```python
from build123d import *

# Parameters (mm, degrees)
SKETCH5_R           = 37.8968
BOSS_EXTRUDE2_DEPTH = 19.05
CUT_EXTRUDE1_DEPTH  = 22.05
CIRPATTERN1_COUNT   = 25
SKETCH9_R           = 7.25
CUT_EXTRUDE2_DEPTH  = 25.4


with BuildPart() as part:
    # Sketch5 → Boss-Extrude2 (new body)
    with BuildSketch(Plane(origin=(0, 0, 0), x_dir=(1, 0, 0), z_dir=(0, 1, 0))):
        with Locations(Location((0, 0, 0), (0, 0, 90))):
            Circle(SKETCH5_R)
    extrude(amount=BOSS_EXTRUDE2_DEPTH)

    # Sketch8 → Cut-Extrude1 (cut)
    with BuildSketch(Plane(origin=(0, 19.05, 0), x_dir=(1, 0, 0), z_dir=(0, 1, 0))):
        Polygon((0, 37.8968), (2.36, 37.8968), (1.66, 35.8968), (0, 35.8968), (-1.66, 35.8968), (-2.36, 37.8968), align=None)
    cut_extrude1 = extrude(amount=-CUT_EXTRUDE1_DEPTH, mode=Mode.SUBTRACT)

    # CirPattern1: Cut-Extrude1 ×25 about axis
    cirpattern1_axis = Axis((0, 0, 0), (0, 1, 0))
    for i in range(1, CIRPATTERN1_COUNT):
        add(cut_extrude1.rotate(cirpattern1_axis, i * 360 / CIRPATTERN1_COUNT), mode=Mode.SUBTRACT)

    # Sketch9 → Cut-Extrude2 (cut)
    with BuildSketch(Plane(origin=(0, 19.05, 0), x_dir=(1, 0, 0), z_dir=(0, 1, 0))):
        Circle(SKETCH9_R)
        Polygon((2.6, 9.75), (2.6, 7.25), (0, 7.25), (-2.6, 7.25), (-2.6, 9.75), align=None)
        with BuildLine():
            ThreePointArc((-2.6, 6.767754428), (-1.32217253, 7.128419166), (0, 7.25))
            Line((0, 7.25), (-2.6, 7.25))
            Line((-2.6, 7.25), (-2.6, 6.767754428))
        make_face()
        with BuildLine():
            Line((2.6, 7.25), (0, 7.25))
            ThreePointArc((0, 7.25), (1.32217253, 7.128419166), (2.6, 6.767754428))
            Line((2.6, 6.767754428), (2.6, 7.25))
        make_face()
    extrude(amount=-CUT_EXTRUDE2_DEPTH, mode=Mode.SUBTRACT)


solid = part.part
```
For this review, take the finished solid that the model builds, in its own axes (mm). A direction names the side the tool comes from. Coordinates: 2 decimals unless noted, no trailing zeros. Order: outer loops, then holes, each group sorted by start corner. A loop starts at its lowest first (then second) coordinate and runs counter-clockwise, first axis right, second up. Notation, with made-up numbers: (41, 57.5) -> (56, 57.5) arc R36 cw to (56, 91.5) -> close; hole circle Ø9 at (76, -1). An arc over 180 degrees is marked (long way). Use CSV: the item, a comma, the result in double quotes. Start each with the question number.
Item 1: Draft analysis for pull direction X (two halves, no side actions). For faces 1 (the face through (-21.081, 9.658, 29.055)), 2 (the face through (-7.23, 9.66, -36.21)), 3 (the face through (-32, 9.4, 20.3)), 4 (the face through (37.82, 9.39, 2.41)), state which applies: pulls with the +X half, pulls with the -X half, needs draft (parallel to the pull), parting line crosses it, or undercut.
Item 2: We need section A-A, the plane x = 0. Give the boundary of the cut face in (y, z).
Item 3: We need section B-B, the plane z = -23.5. Give the boundary of the cut face in (x, y), then the cut area to 3 significant figures.
Item 4: Wall thickness on probe 1 along Z at (x, y) = (0, 10.5); probe 2 along X at (y, z) = (5.25, 0); probe 3 along Z at (x, y) = (3, 13.25): over which ranges is each line inside the solid? List them lowest first.
Item 5: Insertion check: pin 1 (5 mm diameter, centred on y = 16.5, z = 12, fed in from -X); pin 2 (4 mm diameter, centred on x = -1, y = 11, fed in from +Z); pin 3 (1.5 mm diameter, centred on x = 7.5, y = 2.5, fed in from +Z). Each pin has a flat end and moves straight along its axis. Give the tip position at first contact, or say it passes through.
Item 6: For faces 5 (the face through (-26.68, 9.66, -25.5)), 6 (the face through (35.265, 9.658, 6.704)), 7 (the face through (4.783, 9.392, -37.594)), 8 (the face through (9.392, 9.392, 36.715)), 9 (the face through (-36.596, 9.658, 4.943)), list the 3-axis set-ups (+Z, -Z, +X, -X, +Y, -Y) from which the entire face can be reached by the end or side of a thin tool; tool diameter is ignored.
Item 7: We need section C-C, the plane x = 13.5. Give the boundary of the cut face in (y, z), then the cut area to 3 significant figures.
Derived:
1,face 1,"undercut"
1,face 2,"undercut"
1,face 3,"pulls with the -X half"
1,face 4,"pulls with the +X half"
2,outline,"(0, -35.9) -> (19.05, -35.9) -> (19.05, -9.75) -> (0, -9.75) -> close; (0, 7.25) -> (19.05, 7.25) -> (19.05, 37.9) -> (0, 37.9) -> close"
3,outline,"(-29.73, 0) -> (29.73, 0) -> (29.73, 19.05) -> (-29.73, 19.05) -> close"
3,area,"1,130 mm^2"
4,probe 1,"z = -35.9 to -9.75, 7.25 to 37.9"
4,probe 2,"x = -37.9 to -7.25, 7.25 to 37.9"
4,probe 3,"z = -37.78 to -6.6, 6.6 to 35.8"
5,pin 1,"stops at x = -36.69"
5,pin 2,"stops at z = 37.9"
5,pin 3,"stops at z = 37.23"
6,face 5,"-Z, +Y, -Y"
6,face 6,"+X, +Y, -Y"
6,face 7,"-Z, +X, +Y, -Y"
6,face 8,"+Z, +X, +Y, -Y"
6,face 9,"-X, +Y, -Y"
7,outline,"(0, -35.41) -> (19.05, -35.41) -> (19.05, 33.26) -> (0, 33.26) -> close"
7,area,"1,310 mm^2"
